```python
from build123d import *

# Parameters (mm, degrees)
SKETCH1_W           = 42.75
SKETCH1_H           = 30.25
BOSS_EXTRUDE1_DEPTH = 1.5
BOSS_EXTRUDE2_DEPTH = 14
SKETCH3_W           = 2
SKETCH3_H           = 7.6
BOSS_EXTRUDE3_DEPTH = 5
SKETCH4_R           = 2.25
CUT_EXTRUDE1_DEPTH  = 2.5


with BuildPart() as part:
    # Sketch1 → Boss-Extrude1 (new body)
    with BuildSketch(Plane.XY):
        Rectangle(SKETCH1_W, SKETCH1_H)
    extrude(amount=BOSS_EXTRUDE1_DEPTH)

    # Sketch2 → Boss-Extrude2 (add)
    with BuildSketch(Plane(origin=(0, 0, 0), x_dir=(-1, 0, 0), z_dir=(0, 0, -1))):
        Polygon((7.348076211, -13.625), (4.75, -12.125), (-5.25, -12.125), (-7.848076211, -13.625), (-5.25, -15.125), (4.75, -15.125), align=None)
        Polygon((-7.848076211, 13.625), (-5.25, 12.125), (4.75, 12.125), (7.348076211, 13.625), (4.75, 15.125), (-5.25, 15.125), align=None)
    extrude(amount=BOSS_EXTRUDE2_DEPTH)

    # Sketch3 → Boss-Extrude3 (add)
    with BuildSketch(Plane(origin=(0, 0, 0), x_dir=(-1, 0, 0), z_dir=(0, 0, -1))):
        with Locations((20.375, -3.125)):
            Rectangle(SKETCH3_W, SKETCH3_H)
    extrude(amount=BOSS_EXTRUDE3_DEPTH)

    # Sketch4 → Cut-Extrude1 (cut, through all)
    with BuildSketch(Plane(origin=(0, 0, 0), x_dir=(-1, 0, 0), z_dir=(0, 0, -1))):
        with Locations((13.375, 2.125)):
            Circle(SKETCH4_R)
    extrude(amount=-CUT_EXTRUDE1_DEPTH, mode=Mode.SUBTRACT)


solid = part.part
```
Source: CAD feature listing. Evaluate the final solid. Frame: model axes, mm. A direction names the side the tool comes from. Coordinates: 2 decimals unless noted, no trailing zeros. Loops run counter-clockwise (first coordinate to the right, second up) from the corner with the lowest first, then second, coordinate; pieces in that order, holes last. Notation, with made-up numbers: (71, 81.5) -> (118, 81.5) arc R13 ccw to (118, 89.5) -> close; hole circle Ø11 at (-26, -40). An arc over 180 degrees is marked (long way). One line per item, written item: value. Start each with the question number.
Q1. Set-up query: faces 4 (the face through (6.531, 14.386, -6.902)), 5 (the face through (-6.067, -12.886, -6.902)), 6 (the face through (-20, 0.675, -2)), 7 (the face through (6.531, -12.864, -6.902)), 8 (the face through (0, -12.125, -7)). Return all of +Z, -Z, +X, -X, +Y, -Y with unobstructed straight access to the full face (end or side cutting, diameter ignored); none if empty.
Q2. Contact query for flat-ended pins moving along their axis: P1, Ø1.6, axis at x = -20, z = -2, coming from the +Y side (3 decimals); P2, Ø3, axis at x = 10.5, y = -9.5, coming from the -Z side; P3, Ø1.6, axis at x = -20.5, z = -3, coming from the -Y side (3 decimals). Output: stop coordinate, or through.
Q3. Mould query, pull axis Y, two halves, no side actions, for faces 1 (the face through (-6.031, 12.864, -6.902)), 2 (the face through (-6.031, -14.386, -6.902)), 3 (the face through (-21.375, 0, 0)). Classes: pulls with the +Y half, pulls with the -Y half, needs draft (parallel to the pull), parting line crosses it, or undercut.
Q4. Line query: line 1 along Y through (x, z) = (2, -10.5) (3 decimals); line 2 along Z through (x, y) = (-5, -8); line 3 along Y through (x, z) = (-6.5, -10.25). Output: solid intervals per line, ascending.
Q5. Section query C-C, the plane x = 2.5. Return the cut outline in (y, z) (3 decimals), and give its area (3 significant figures).
Q6. Section query D-D, the plane y = -2.5. Return the cut outline in (x, z) (3 decimals).
Q7. Section query A-A, the plane z = -0.5. Return the cut outline in (x, y) (3 decimals).
Q8. Section query B-B, the plane z = -9.25. Return the cut outline in (x, y) (3 decimals).
Results:
1. face 4: -Z, +X, +Y
1. face 5: -Z, -X
1. face 6: -Z, +X, -X, +Y
1. face 7: -Z, +X
1. face 8: -Z, +X, -X
2. P1: y = 0.675
2. P2: z = 0
2. P3: y = -6.925
3. face 1: undercut
3. face 2: pulls with the -Y half
3. face 3: needs draft
4. line 1: -15.125 to -12.125, 12.125 to 15.125
4. line 2: 0 to 1.5
4. line 3: -14.11 to -13.14, 13.14 to 14.11
5. outline: (-15.125, -14) -> (-12.125, -14) -> (-12.125, 0) -> (12.125, 0) -> (12.125, -14) -> (15.125, -14) -> (15.125, 1.5) -> (-15.125, 1.5) -> close
5. area: 129 mm^2
6. outline: (-21.375, -5) -> (-19.375, -5) -> (-19.375, 0) -> (21.375, 0) -> (21.375, 1.5) -> (-21.375, 1.5) -> close
7. outline: (-21.375, -6.925) -> (-19.375, -6.925) -> (-19.375, 0.675) -> (-21.375, 0.675) -> close; (-7.348, -13.625) -> (-4.75, -15.125) -> (5.25, -15.125) -> (7.848, -13.625) -> (5.25, -12.125) -> (-4.75, -12.125) -> close; (-7.348, 13.625) -> (-4.75, 12.125) -> (5.25, 12.125) -> (7.848, 13.625) -> (5.25, 15.125) -> (-4.75, 15.125) -> close
8. outline: (-7.348, -13.625) -> (-4.75, -15.125) -> (5.25, -15.125) -> (7.848, -13.625) -> (5.25, -12.125) -> (-4.75, -12.125) -> close; (-7.348, 13.625) -> (-4.75, 12.125) -> (5.25, 12.125) -> (7.848, 13.625) -> (5.25, 15.125) -> (-4.75, 15.125) -> close
